Here's how the part is built. I have some questions about the finished solid (model axes, mm). Round coordinates to 2 decimals unless told otherwise and drop trailing zeros. Order: outer loops, then holes, each group sorted by start corner. A loop starts at its lowest first (then second) coordinate and runs counter-clockwise, first axis right, second up. Notation, with made-up numbers: M -1,17.5 L 18,17.5 A23 cw 18,36.5 Z; hole C -13.5,41.5 d11. An arc over 180 degrees is marked long. Write item = value, one per line. Start each with the question number.
Item 1: I'm going to push flat-ended pins straight in: P1, Ø1.4, axis at x = 52.5, y = 2.5, coming from the -Z side; P2, Ø1.4, axis at x = 31, y = 1.5, coming from the +Z side. Where does each tip first touch, or does it pass through?
Item 2: I want a section at A-A, the plane x = 38.5. List the corners of the cut face in (y, z) for me.
Item 3: Please list where these lines run through material, in increasing order: L1, parallel to X at y = 2.55, z = 42; L2, parallel to X at y = 2.2, z = -113.5; L3, parallel to Z at x = 34, y = 0.6.
Item 4: I want a section at C-C, the plane z = -36.5. List the corners of the cut face in (x, y) for me, plus the area to 3 significant figures.
Item 5: I want a section at B-B, the plane y = 4. State how many separate pieces and enclosed holes the cut face has, plus the area to 3 significant figures.
```python
from build123d import *

# Parameters (mm, degrees)
SKETCH1_W                 = 203.2
SKETCH1_H                 = 330.2
BASE_DEPTH                = 4.7625
HOLES_DEPTH               = 194.915578039
HOLES_DEPTH_BACK          = 194.915578039
SKETCH2_R                 = 3.302
SUS_TAB_CUTOUT_DEPTH      = 194.915578039
SUS_TAB_CUTOUT_DEPTH_BACK = 194.915578039
SKETCH3_W                 = 104.14
SKETCH3_H                 = 25.4
INNER_CUTOUT_DEPTH        = 194.915578039
INNER_CUTOUT_DEPTH_BACK   = 194.915578039
FILLET1_R                 = 6.35
FILLET2_R                 = 12.7


with BuildPart() as part:
    # Sketch1 → Base (new body)
    with BuildSketch(Plane(origin=(0, 0, 0), x_dir=(1, 0, 0), z_dir=(0, 1, 0))):
        Rectangle(SKETCH1_W, SKETCH1_H)
    extrude(amount=BASE_DEPTH)

    # Sketch2 → Holes (cut, two sides: drawn at the far end of the back side and taken through both)
    with BuildSketch(Plane(origin=(0, 4.7625, 0), x_dir=(1, 0, 0), z_dir=(0, 1, 0)).offset(-HOLES_DEPTH_BACK)):
        with Locations(Location((-88.9, 139.7, 0), (0, 0, 270))):
            Circle(SKETCH2_R)
        with Locations(Location((-88.9, -139.7, 0), (0, 0, 270))):
            Circle(SKETCH2_R)
        with Locations(Location((88.9, -127, 0), (0, 0, 270))):
            Circle(SKETCH2_R)
        with Locations(Location((88.9, 127, 0), (0, 0, 270))):
            Circle(SKETCH2_R)
    extrude(amount=HOLES_DEPTH + HOLES_DEPTH_BACK, mode=Mode.SUBTRACT)

    # Sketch3 → Sus Tab Cutout (cut, two sides: drawn at the far end of the back side and taken through both)
    with BuildSketch(Plane(origin=(0, 4.7625, 0), x_dir=(1, 0, 0), z_dir=(0, 1, 0)).offset(-SUS_TAB_CUTOUT_DEPTH_BACK)):
        with Locations((49.53, 152.4)):
            Rectangle(SKETCH3_W, SKETCH3_H)
        with Locations((49.53, -152.4)):
            Rectangle(SKETCH3_W, SKETCH3_H)
    extrude(amount=SUS_TAB_CUTOUT_DEPTH + SUS_TAB_CUTOUT_DEPTH_BACK, mode=Mode.SUBTRACT)

    # Sketch4 → Inner Cutout (cut, two sides: drawn at the far end of the back side and taken through both)
    with BuildSketch(Plane(origin=(0, 4.7625, 0), x_dir=(1, 0, 0), z_dir=(0, 1, 0)).offset(-INNER_CUTOUT_DEPTH_BACK)):
        with BuildLine():
            Line((88.9, 114.3), (88.9, -114.3))
            ThreePointArc((88.9, -114.3), (79.919743879, -118.019743879), (76.2, -127))
            Line((76.2, -127), (-88.9, -127))
            Line((-88.9, -127), (-88.9, 127))
            Line((-88.9, 127), (76.2, 127))
            ThreePointArc((76.2, 127), (79.919743879, 118.019743879), (88.9, 114.3))
        make_face()
    extrude(amount=INNER_CUTOUT_DEPTH + INNER_CUTOUT_DEPTH_BACK, mode=Mode.SUBTRACT)

    # Fillet1
    fillet1_edges = [part.edges().sort_by_distance(p)[0] for p in [
        (-2.54, 2.38125, -165.1),
        (101.6, 2.38125, -139.7),
        (-2.54, 2.38125, -139.7),
        (-2.54, 2.38125, 165.1),
        (-2.54, 2.38125, 139.7),
        (101.6, 2.38125, 139.7),
        (-101.6, 2.38125, 165.1),
        (-101.6, 2.38125, -165.1),
    ]]
    fillet(fillet1_edges, radius=FILLET1_R)

    # Fillet2
    fillet2_edges = [part.edges().sort_by_distance(p)[0] for p in [
        (-88.9, 2.38125, -127),
        (76.2, 2.38125, -127),
        (88.9, 2.38125, -114.3),
        (88.9, 2.38125, 114.3),
        (76.2, 2.38125, 127),
        (-88.9, 2.38125, 127),
    ]]
    fillet(fillet2_edges, radius=FILLET2_R)


solid = part.part
```
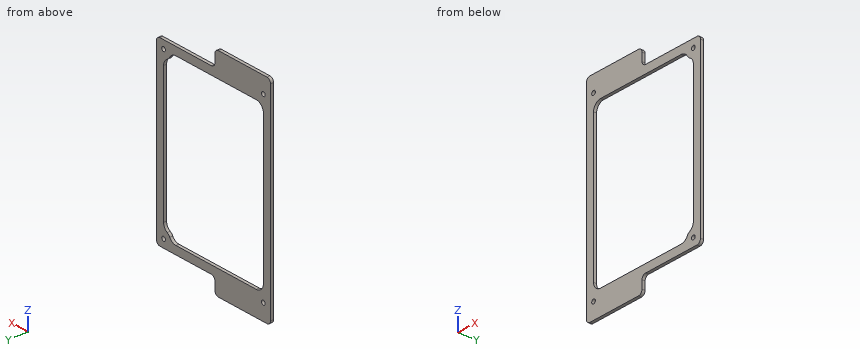
Filled in:
q1.P1 = -139.7
q1.P2 = 139.7
q2.outline = M 0,-139.7 L 4.76,-139.7 L 4.76,-127 L 0,-127 Z; M 0,127 L 4.76,127 L 4.76,139.7 L 0,139.7 Z
q3.L1 = -101.6 to -88.9, 88.9 to 101.6
q3.L2 = -101.6 to -88.9, 85.64 to 101.6
q3.L3 = -139.7 to -127, 127 to 139.7
q4.outline = M -101.6,0 L -88.9,0 L -88.9,4.76 L -101.6,4.76 Z; M 88.9,0 L 101.6,0 L 101.6,4.76 L 88.9,4.76 Z
q4.area = 121 mm^2
q5.separate_pieces = 1
q5.enclosed_holes = 5
q5.area = 16,800 mm^2
